Check sheet for the modelled part. Datum: model origin and axes. Units: mm. Face numbers are marked on the shaded views. A direction names the side the tool comes from. Coordinates: 2 decimals unless noted, no trailing zeros. Write each loop counter-clockwise with the first axis right and the second up, starting at its lowest first coordinate (ties: lowest second). Pieces come first, ordered by that corner, then holes. Notation, with made-up numbers: (24, 68.5) - (77, 68.5) arc R34 ccw to (77, 106.5) - close; hole circle Ø11 at (57, 24). An arc over 180 degrees is marked (long way). Use one line per item in the form item = value. Start each with the question number.
1. Cross-section at D-D on y = 5.5. Record the boundary of the cut face in (x, z), then the cut area to 3 significant figures.
2. Tool access check on the marked faces 1 and 2. Record the directions out of +Z, -Z, +X, -X, +Y, -Y that give a thin tool (end or side, any length) a straight path to the whole face; none if there is none.
3. Draft check along Y on the marked faces 3, 4 and 5. Enter one of: +Y half, -Y half, draft (parallel to the pull), parting line (faces both ways), or undercut.
4. Scan lines: line 1 along Y through (x, z) = (-2.25, 7); line 2 along X through (y, z) = (-5.5, 6.25); line 3 along X through (y, z) = (0.75, 5.5). Record each from-to range of solid material in increasing order.
5. Cross-section at B-B on x = 0. Record the boundary of the cut face in (y, z), then the cut area to 3 significant figures.
6. Cross-section at C-C on y = 0. Record the boundary of the cut face in (x, z).
7. Cross-section at A-A on z = 7.5. Record the boundary of the cut face in (x, y), then the cut area to 3 significant figures.
8. Go/stop test with flat-tipped pins: pin 1 Ø2.5 at (y, z) = (-1.5, 8) entering from -X; pin 2 Ø4 at (y, z) = (-3.5, 4) entering from -X; pin 3 Ø3 at (x, z) = (5, 7) entering from +Y. Record where each tip stops, or that it passes through.
```python
from build123d import *

# Parameters (mm, degrees)
SKETCH2_R           = 12
BOSS_EXTRUDE1_DEPTH = 12
CUT_EXTRUDE1_DEPTH  = 10


with BuildPart() as part:
    # Sketch2 → Boss-Extrude1 (new body)
    with BuildSketch(Plane.XY):
        Circle(SKETCH2_R)
    extrude(amount=BOSS_EXTRUDE1_DEPTH)

    # Sketch3 → Cut-Extrude1 (cut)
    with BuildSketch(Plane.XY.offset(12)):
        Polygon((3.581048399, -4.334317157), (7.028622417, -4.334317157), (7.028622417, 4.334317157), (-7.028622417, 4.334317157), (-7.028622417, -4.334317157), (-3.581048399, -4.334317157), (-3.581048399, -5.807105512), (-1.439194114, -5.807105512), (-1.439194114, -6.576782405), (1.439194114, -6.576782405), (1.439194114, -5.807105512), (3.581048399, -5.807105512), align=None)
    extrude(amount=-CUT_EXTRUDE1_DEPTH, mode=Mode.SUBTRACT)


solid = part.part
```
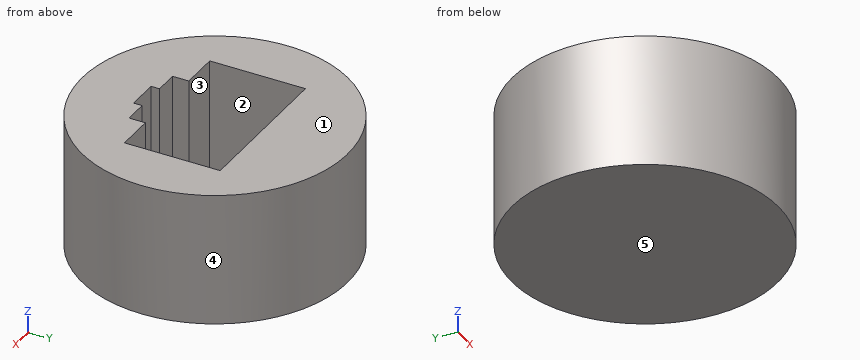
Final values:
q1.outline = (-10.67, 0) - (10.67, 0) - (10.67, 12) - (-10.67, 12) - close
q1.area = 256 mm²
q2.face_1 = +Z, +X, -X, +Y, -Y
q2.face_2 = +Z
q3.face_3 = undercut
q3.face_4 = parting line
q3.face_5 = draft
q4.line_1 = -11.79 to -5.81, 4.33 to 11.79
q4.line_2 = -10.67 to -3.58, 3.58 to 10.67
q4.line_3 = -11.98 to -7.03, 7.03 to 11.98
q5.outline = (-12, 0) - (12, 0) - (12, 12) - (4.33, 12) - (4.33, 2) - (-6.58, 2) - (-6.58, 12) - (-12, 12) - close
q5.area = 179 mm²
q6.outline = (-12, 0) - (12, 0) - (12, 12) - (7.03, 12) - (7.03, 2) - (-7.03, 2) - (-7.03, 12) - (-12, 12) - close
q7.outline = circle Ø24 at (0, 0); hole (-7.03, -4.33) - (-3.58, -4.33) - (-3.58, -5.81) - (-1.44, -5.81) - (-1.44, -6.58) - (1.44, -6.58) - (1.44, -5.81) - (3.58, -5.81) - (3.58, -4.33) - (7.03, -4.33) - (7.03, 4.33) - (-7.03, 4.33) - close
q7.area = 318 mm²
q8.pin_1 = -12
q8.pin_2 = -11.91
q8.pin_3 = 11.48
